from build123d import *

# Parameters (mm, degrees)
SKETCH2_R           = 1.5
BOSS_EXTRUDE4_DEPTH = 3


with BuildPart() as part:
    # Sketch2 → Boss-Extrude4 (new body)
    with BuildSketch(Plane.XY.offset(-649.589603716)):
        with BuildLine():
            Line((40.97386422, 223.853671966), (-49.02613578, 223.853671966))
            ThreePointArc((-49.02613578, 223.853671966), (-57.157863764, 220.48539995), (-60.52613578, 212.353671966))
            Line((-60.52613578, 212.353671966), (-60.52613578, 117.353671966))
            ThreePointArc((-60.52613578, 117.353671966), (-58.622329858, 112.757477888), (-54.02613578, 110.853671966))
            Line((-54.02613578, 110.853671966), (45.97386422, 110.853671966))
            ThreePointArc((45.97386422, 110.853671966), (50.570058297, 112.757477888), (52.47386422, 117.353671966))
            Line((52.47386422, 117.353671966), (52.47386422, 212.353671966))
            ThreePointArc((52.47386422, 212.353671966), (49.105592203, 220.48539995), (40.97386422, 223.853671966))
        make_face()
        with Locations((-56.02613578, 201.353671966)):
            Circle(SKETCH2_R, mode=Mode.SUBTRACT)
        with Locations((-24.02613578, 219.356652382)):
            Circle(SKETCH2_R, mode=Mode.SUBTRACT)
        with Locations((15.97386422, 219.356652382)):
            Circle(SKETCH2_R, mode=Mode.SUBTRACT)
        with Locations((47.97386422, 201.353671966)):
            Circle(SKETCH2_R, mode=Mode.SUBTRACT)
        with Locations((47.97386422, 140.353671966)):
            Circle(SKETCH2_R, mode=Mode.SUBTRACT)
        with Locations((-56.02613578, 140.353671966)):
            Circle(SKETCH2_R, mode=Mode.SUBTRACT)
        with BuildLine():
            Line((-53.02613578, 192.353671966), (-53.02613578, 162.353671966))
            Line((-53.02613578, 162.353671966), (-53.02613578, 149.353671966))
            ThreePointArc((-53.02613578, 149.353671966), (-52.490237396, 147.353671966), (-51.02613578, 145.889570351))
            ThreePointArc((-51.02613578, 145.889570351), (-49.562034165, 144.425468736), (-49.02613578, 142.425468736))
            Line((-49.02613578, 142.425468736), (-49.02613578, 134.353671966))
            ThreePointArc((-49.02613578, 134.353671966), (-47.854562905, 131.525244841), (-45.02613578, 130.353671966))
            Line((-45.02613578, 130.353671966), (36.97386422, 130.353671966))
            ThreePointArc((36.97386422, 130.353671966), (39.802291344, 131.525244841), (40.97386422, 134.353671966))
            Line((40.97386422, 134.353671966), (40.97386422, 142.425468736))
            ThreePointArc((40.97386422, 142.425468736), (41.509762604, 144.425468736), (42.97386422, 145.889570351))
            ThreePointArc((42.97386422, 145.889570351), (44.437965835, 147.353671966), (44.97386422, 149.353671966))
            Line((44.97386422, 149.353671966), (44.97386422, 192.353671966))
            ThreePointArc((44.97386422, 192.353671966), (44.437965835, 194.353671966), (42.97386422, 195.817773581))
            ThreePointArc((42.97386422, 195.817773581), (41.509762604, 197.281875196), (40.97386422, 199.281875196))
            Line((40.97386422, 199.281875196), (40.97386422, 203.425468736))
            ThreePointArc((40.97386422, 203.425468736), (41.509762604, 205.425468736), (42.97386422, 206.889570351))
            ThreePointArc((42.97386422, 206.889570351), (44.437965835, 208.353671966), (44.97386422, 210.353671966))
            Line((44.97386422, 210.353671966), (44.97386422, 212.353671966))
            ThreePointArc((44.97386422, 212.353671966), (43.802291344, 215.182099091), (40.97386422, 216.353671966))
            Line((40.97386422, 216.353671966), (24.97386422, 216.353671966))
            ThreePointArc((24.97386422, 216.353671966), (22.97386422, 215.817773581), (21.509762604, 214.353671966))
            ThreePointArc((21.509762604, 214.353671966), (20.045660989, 212.889570351), (18.045660989, 212.353671966))
            Line((18.045660989, 212.353671966), (13.90206745, 212.353671966))
            ThreePointArc((13.90206745, 212.353671966), (11.90206745, 212.889570351), (10.437965835, 214.353671966))
            ThreePointArc((10.437965835, 214.353671966), (8.97386422, 215.817773581), (6.97386422, 216.353671966))
            Line((6.97386422, 216.353671966), (-15.02613578, 216.353671966))
            ThreePointArc((-15.02613578, 216.353671966), (-17.02613578, 215.817773581), (-18.490237396, 214.353671966))
            ThreePointArc((-18.490237396, 214.353671966), (-19.954339011, 212.889570351), (-21.954339011, 212.353671966))
            Line((-21.954339011, 212.353671966), (-26.09793255, 212.353671966))
            ThreePointArc((-26.09793255, 212.353671966), (-28.09793255, 212.889570351), (-29.562034165, 214.353671966))
            ThreePointArc((-29.562034165, 214.353671966), (-31.02613578, 215.817773581), (-33.02613578, 216.353671966))
            Line((-33.02613578, 216.353671966), (-49.02613578, 216.353671966))
            ThreePointArc((-49.02613578, 216.353671966), (-51.854562905, 215.182099091), (-53.02613578, 212.353671966))
            Line((-53.02613578, 212.353671966), (-53.02613578, 210.353671966))
            ThreePointArc((-53.02613578, 210.353671966), (-52.490237396, 208.353671966), (-51.02613578, 206.889570351))
            ThreePointArc((-51.02613578, 206.889570351), (-49.562034165, 205.425468736), (-49.02613578, 203.425468736))
            Line((-49.02613578, 203.425468736), (-49.02613578, 199.281875196))
            ThreePointArc((-49.02613578, 199.281875196), (-49.562034165, 197.281875196), (-51.02613578, 195.817773581))
            ThreePointArc((-51.02613578, 195.817773581), (-52.490237396, 194.353671966), (-53.02613578, 192.353671966))
        make_face(mode=Mode.SUBTRACT)
    extrude(amount=BOSS_EXTRUDE4_DEPTH)


solid = part.part
Geometry: final body of the model. Coordinates: model frame, mm. A direction names the side the tool comes from. Coordinates: 2 decimals unless noted, no trailing zeros. Loops run counter-clockwise (first coordinate to the right, second up) from the corner with the lowest first, then second, coordinate; pieces in that order, holes last. Notation, with made-up numbers: (1.25, 29.25) - (21.25, 29.25) arc R13 ccw to (21.25, 47.25) - close; hole circle Ø3 at (-29.5, -18.75). An arc over 180 degrees is marked (long way). One line per question, with ' | ' between items. Start each with the question number.
(1) Cut plane A-A on y = 151. Output: boundary loops of the cut face in (x, z).
(2) Cut plane B-B on x = -2. Output: boundary loops of the cut face in (y, z).
(3) Ray query, L1, parallel to Y at x = 33, z = -647.7; L2, parallel to X at y = 160.5, z = -648; L3, parallel to Y at x = 48.5, z = -647.3. Return the intervals inside material, ascending. Write a range as from..to.
(4) Draft query along X for faces 3 (the flat face through (-41, 216.354, -648)), 4 (the flat face through (52.474, 164, -648)), 5 (the flat face through (-55, 168, -649.59)). Return one class per face: +X half, -X half, draft (parallel to the pull), parting line (faces both ways), or undercut.
(5) Cut plane C-C on z = -647.95. Count the separate pieces of the cut face and the enclosed holes in it, and give its area (3 significant figures).
(6) First-contact query: pin 1 (1.5 mm diameter, centred on x = 39.5, y = 137.5, fed in from +Z) (1 decimal); pin 2 (5 mm diameter, centred on x = -56.03, y = 140.35, fed in from +Z). Flat tips, straight axial feed; report the tip coordinate or a pass-through.
(7) Reachability of faces 1 (the cylindrical face through (-58.673, 112.808, -648.111)), 2 (the flat face through (-49.026, 201, -648)) from +Z, -Z, +X, -X, +Y, -Y: full face, straight path, thin tool, end or side. Return the list, or none.
Here are the results:
1) outline: (-60.53, -649.59) - (-53.03, -649.59) - (-53.03, -646.59) - (-60.53, -646.59) - close; (44.97, -649.59) - (52.47, -649.59) - (52.47, -646.59) - (44.97, -646.59) - close
2) outline: (110.85, -649.59) - (130.35, -649.59) - (130.35, -646.59) - (110.85, -646.59) - close; (216.35, -649.59) - (223.85, -649.59) - (223.85, -646.59) - (216.35, -646.59) - close
3) L1: 110.85..130.35, 216.35..223.85 | L2: -60.53..-53.03, 44.97..52.47 | L3: 111.36..138.95, 141.76..199.95, 202.76..221.05
4) face 3: undercut | face 4: +X half | face 5: draft
5) separate pieces: 1 | enclosed holes: 7 | area: 4,540 mm²
6) pin 1: through | pin 2: z = -646.59
7) face 1: +Z, -Z, -X, -Y | face 2: +Z, -Z
